The model under review builds one solid part; all positions refer to its coordinate system, in mm. A direction names the side the tool comes from. Coordinates: 2 decimals unless noted, no trailing zeros. Write each loop counter-clockwise with the first axis right and the second up, starting at its lowest first coordinate (ties: lowest second). Pieces come first, ordered by that corner, then holes. Notation, with made-up numbers: (76, 74) - (107, 74) arc R26 ccw to (107, 110) - close; hole circle Ø10 at (34, -24.75). An arc over 180 degrees is marked (long way). Return JSON: item names as keys, results as strings. Group by question number.
(1) For pin 1 Ø5 at (x, y) = (-14, 12.5) entering from +Z; pin 2 Ø5 at (y, z) = (21.5, 15) entering from -X; pin 3 Ø3 at (x, z) = (-1.5, 6.5) entering from -Y; pin 4 Ø1.5 at (x, z) = (10.5, 9.5) entering from +Y, all flat-tipped, find the tip position at first contact; note any pin that passes through.
(2) We need section B-B on y = 147.5. State the section outline as (x, z) points.
(3) To check wall thickness, follow L1, parallel to Y at x = -4, z = 8; L2, parallel to X at y = -68.5, z = 11.25; L3, parallel to Z at x = -12.5, y = -72. State the ranges of each line that lie inside material, in increasing order. Write a range as from..to.
(4) We need section A-A on x = 4.5. State the section outline as (y, z) points, then the cut area to 3 significant figures.
(5) Tool access review of faces 1 (the face through (-10, -3, 15)), 2 (the face through (5, 185, 10)), 3 (the face through (5, -190, 15)), 4 (the face through (0, 3, 0)), 5 (the face through (5, -185, 10)): name each direction out of +Z, -Z, +X, -X, +Y, -Y from which nothing blocks a thin tool from reaching the whole face with its end or side.
(6) We need section C-C on z = 13.5. State the section outline as (x, y) points, then the cut area to 3 significant figures.
(7) We need section D-D on x = -15. State the section outline as (y, z) points, then the cut area to 3 significant figures.
```python
from build123d import *

# Parameters (mm, degrees)
SKETCH1_W           = 40
SKETCH1_H           = 380
BOSS_EXTRUDE1_DEPTH = 20
SKETCH2_W           = 10
SKETCH2_H           = 380
CUT_EXTRUDE1_DEPTH  = 10
SKETCH3_W           = 40
SKETCH3_H           = 10
CUT_EXTRUDE2_DEPTH  = 10


with BuildPart() as part:
    # Sketch1 → Boss-Extrude1 (new body)
    with BuildSketch(Plane.XY):
        Rectangle(SKETCH1_W, SKETCH1_H)
    extrude(amount=BOSS_EXTRUDE1_DEPTH)

    # Sketch2 → Cut-Extrude1 (cut)
    with BuildSketch(Plane.XY.offset(20)):
        with Locations((-15, 0)):
            Rectangle(SKETCH2_W, SKETCH2_H)
    extrude(amount=-CUT_EXTRUDE1_DEPTH, mode=Mode.SUBTRACT)

    # Sketch3 → Cut-Extrude2 (cut)
    with BuildSketch(Plane(origin=(0, 0, 0), x_dir=(-1, 0, 0), z_dir=(0, 0, -1))):
        with Locations((0, 185)):
            Rectangle(SKETCH3_W, SKETCH3_H)
        with Locations((0, -185)):
            Rectangle(SKETCH3_W, SKETCH3_H)
    extrude(amount=-CUT_EXTRUDE2_DEPTH, mode=Mode.SUBTRACT)


solid = part.part
```
Ans:
{
 "1": {"pin 1": "z = 10", "pin 2": "x = -10", "pin 3": "y = -180", "pin 4": "y = 190"},
 "2": {"outline": "(-20, 0) - (20, 0) - (20, 20) - (-10, 20) - (-10, 10) - (-20, 10) - close"},
 "3": {"L1": "-180..180", "L2": "-10..20", "L3": "0..10"},
 "4": {"outline": "(-190, 10) - (-180, 10) - (-180, 0) - (180, 0) - (180, 10) - (190, 10) - (190, 20) - (-190, 20) - close", "area": "7,400 mm²"},
 "5": {"face 1": "+Z, -X, +Y, -Y", "face 2": "-Z, +X, -X, +Y", "face 3": "+Z, -Z, +X, -X, -Y", "face 4": "-Z, +X, -X, +Y, -Y", "face 5": "-Z, +X, -X, -Y"},
 "6": {"outline": "(-10, -190) - (20, -190) - (20, 190) - (-10, 190) - close", "area": "11,400 mm²"},
 "7": {"outline": "(-180, 0) - (180, 0) - (180, 10) - (-180, 10) - close", "area": "3,600 mm²"}
}
